CAD build for the part. Positions are in the model's coordinates, mm. Face numbers are marked on the shaded views. A direction names the side the tool comes from. Give positions to 0.01 mm unless a question says otherwise; leave off trailing zeros. Loops run counter-clockwise (first coordinate to the right, second up) from the corner with the lowest first, then second, coordinate; pieces in that order, holes last.
```python
from build123d import *

# Parameters (mm, degrees)
F0_W     = 49.773663
F0_H     = 49.463548
F1_DEPTH = 7.62
F2_T     = -1.27
F4_DEPTH = 5.08
F3_W     = 10.467866
F3_H     = 2.113704
F3_R     = 2.24296
F5_DEPTH = 5.08
F6_R     = 1.943924
F7_DEPTH = 5.08


with BuildPart() as f1:
    # F0 (on Top) → F1 (new body)
    with BuildSketch(Plane.XY):
        with Locations((-24.886831, 24.731774)):
            Rectangle(F0_W, F0_H)
    extrude(amount=F1_DEPTH)

    # F2
    f2_openings = [f1.faces().sort_by_distance(p)[0] for p in [
        (-24.886832, 24.731774, 7.62),
    ]]
    offset(amount=F2_T, openings=f2_openings)

    # F3 (on face) → F4 (join)
    with BuildSketch(Plane.XY.offset(1.27)):
        Polygon((-42.308204, 31.621417), (-42.308204, 1.27), (-40.409051, 1.27), (-40.409051, 30.519297), (-40.409051, 31.621417), align=None)
    extrude(amount=F4_DEPTH)

    # F3 (on face) → F5 (join)
    with BuildSketch(Plane.XY.offset(1.27)):
        Polygon((-42.308204, 31.621417), (-42.308204, 1.27), (-40.409051, 1.27), (-40.409051, 30.519297), (-40.409051, 31.621417), align=None)
        Polygon((-40.409051, 31.621417), (-40.409051, 30.519297), (-30.573701, 30.519297), (-30.573701, 31.621417), (-32.687407, 31.621417), align=None)
        Polygon((-32.687407, 43.805435), (-32.687407, 31.621417), (-30.573701, 31.621417), (-30.573701, 39.980639), (-30.573701, 41.591078), (-30.573701, 43.805435), align=None)
        Polygon((-30.573701, 41.591078), (-30.573701, 39.980639), (-18.797351, 39.980639), (-16.985605, 39.980639), (-16.985605, 41.591078), align=None)
        Polygon((-16.985605, 39.980639), (-18.797351, 39.980639), (-18.797351, 27.298415), (-16.985605, 27.298415), (-16.985605, 33.639527), (-16.985605, 35.753231), align=None)
        with Locations((-11.751672, 34.696379)):
            Rectangle(F3_W, F3_H)
        with Locations((-42.652011, 39.879985)):
            Circle(F3_R)
    extrude(amount=F5_DEPTH)

    # F6 (on face) → F7 (cut)
    with BuildSketch(Plane.XY.offset(1.27)):
        with Locations((-45.369629, 6.563986)):
            Circle(F6_R)
    extrude(amount=-F7_DEPTH, mode=Mode.SUBTRACT)


solid = f1.part
```
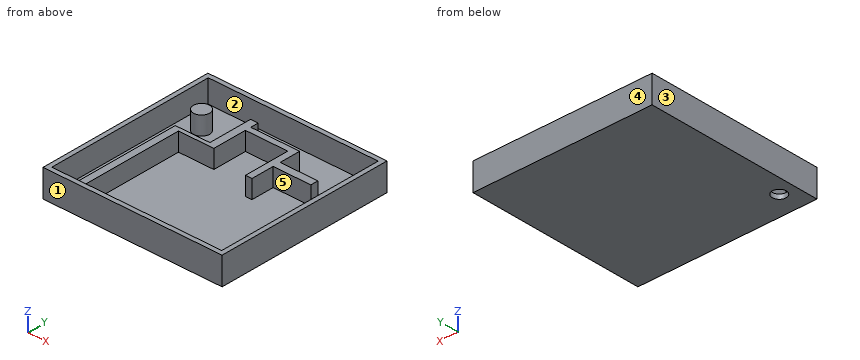
1. Saw through at C-C, the plane z = 3.75. List the corners of the cut face in (x, y), and give its area (3 significant figures).
Responses:
outline: (-49.77, 0) - (0, 0) - (0, 49.46) - (-49.77, 49.46) - close; circle Ø4.49 at (-42.65, 39.88); hole (-48.5, 1.27) - (-42.31, 1.27) - (-42.31, 31.62) - (-32.69, 31.62) - (-32.69, 43.81) - (-30.57, 43.81) - (-30.57, 41.59) - (-16.99, 41.59) - (-16.99, 35.75) - (-6.52, 35.75) - (-6.52, 33.64) - (-16.99, 33.64) - (-16.99, 27.3) - (-18.8, 27.3) - (-18.8, 39.98) - (-30.57, 39.98) - (-30.57, 30.52) - (-40.41, 30.52) - (-40.41, 1.27) - (-1.27, 1.27) - (-1.27, 48.19) - (-48.5, 48.19) - close
area: 423 mm2
2. Saw through at D-D, the plane x = -24. List the corners of the cut face in (y, z), and give its area (3 significant figures).
Responses:
outline: (0, 0) - (49.46, 0) - (49.46, 7.62) - (48.19, 7.62) - (48.19, 1.27) - (41.59, 1.27) - (41.59, 6.35) - (39.98, 6.35) - (39.98, 1.27) - (1.27, 1.27) - (1.27, 7.62) - (0, 7.62) - close
area: 87.1 mm2
3. Saw through at A-A, the plane y = 14. List the corners of the cut face in (x, z).
Responses:
outline: (-49.77, 0) - (0, 0) - (0, 7.62) - (-1.27, 7.62) - (-1.27, 1.27) - (-40.41, 1.27) - (-40.41, 6.35) - (-42.31, 6.35) - (-42.31, 1.27) - (-48.5, 1.27) - (-48.5, 7.62) - (-49.77, 7.62) - close
4. Drop flat-ended pins along their axis: pin 1 (6 mm diameter, centred on x = -21, y = 26.5, fed in from -Z); pin 2 (10 mm diameter, centred on x = -26, y = 29, fed in from +Z); pin 3 (10.5 mm diameter, centred on x = -23, y = 23, fed in from +Z); pin 4 (2.5 mm diameter, centred on x = -45.37, y = 6.56, fed in from +Z). Give the stop position or say it passes through.
Responses:
pin 1: stops at z = 0
pin 2: stops at z = 6.35
pin 3: stops at z = 1.27
pin 4: passes through
5. Tool access for the marked faces 1 and 2: list every direction of +Z, -Z, +X, -X, +Y, -Y with a clear straight run to the whole face (end or side of a thin tool).
Responses:
face 1: +Z, -Z, +X, -X, -Y
face 2: +Z
6. Saw through at B-B, the plane x = -46. List the corners of the cut face in (y, z).
Responses:
outline: (0, 0) - (4.73, 0) - (4.73, 1.27) - (1.27, 1.27) - (1.27, 7.62) - (0, 7.62) - close; (8.4, 0) - (49.46, 0) - (49.46, 7.62) - (48.19, 7.62) - (48.19, 1.27) - (8.4, 1.27) - close
7. Probe line 1 along X through (y, z) = (13.5, 5.5); line 2 along Y through (x, z) = (-20.5, 6.25); line 3 along Y through (x, z) = (-32, 3.75). List the from-to ranges inside material, lowest first.
Responses:
line 1: x = -49.77 to -48.5, -42.31 to -40.41, -1.27 to 0
line 2: y = 0 to 1.27, 39.98 to 41.59, 48.19 to 49.46
line 3: y = 0 to 1.27, 30.52 to 43.81, 48.19 to 49.46
8. Pull direction X, two halves, no side cores. Call the marked faces 3, 4 and 5: released by +X, released by -X, zero draft, split by the parting line, or undercut.
Responses:
face 3: released by -X
face 4: zero draft
face 5: undercut
